Here's how the part is built. I have some questions about the finished solid (model axes, mm). Coordinates: 2 decimals unless noted, no trailing zeros. Loops run counter-clockwise (first coordinate to the right, second up) from the corner with the lowest first, then second, coordinate; pieces in that order, holes last. Notation, with made-up numbers: (53.25, 71) - (79.25, 71) arc R29 ccw to (79.25, 107) - close; hole circle Ø2 at (77, -3). An arc over 180 degrees is marked (long way). Use a Markdown table: item, result.
Autodesk Inventor part; units mm, degrees
ref_plane "YZ Plane" through (0, 0, 0) normal (1, 0, 0) x (0, 1, 0)
ref_plane "XZ Plane" through (0, 0, 0) normal (0, 1, 0) x (-1, 0, 0)
ref_plane "XY Plane" through (0, 0, 0) normal (0, 0, 1) x (1, 0, 0)
sketch "Sketch1" plane through (0, 0, 0) normal (0, 1, 0) x (-1, 0, 0)
  line L0 (25.8082, 8) -> (28.6076, 7.9624) construction
  line L1 (0, 0) -> (0, 92.83)
  line L2 (0, 0) -> (12.1, 0)
  line L3 (26.34, 81.33) -> (8, 81.33)
  line L4 (8, 81.33) -> (8, 32)
  line L5 (8, 32) -> (26.34, 32)
  line L6 (26.34, 32) -> (26.34, 81.33)
  line L7 (0, 92.83) -> (7.42, 92.83)
  line L8 (7.42, 92.83) -> (7.42, 89.33)
  line L9 (7.42, 89.33) -> (26.92, 89.33)
  line L10 (26.92, 89.33) -> (26.92, 92.83)
  line L11 (26.92, 92.83) -> (34.34, 92.83)
  line L12 (34.34, 92.83) -> (34.34, 0)
  line L13 (34.34, 0) -> (12.1, 0)
  line L14 (12.1, 0) -> (12.1, 8)
  line L15 (12.1, 8) -> (34.34, 8)
  spline S0 degree 3 poles (25.8082, 8) (28.6076, 7.9624) (34.5101, 18.742) (34.34, 45.0104) knots 1 1 1 1 1.641396 1.641396 1.641396 1.641396
  line L16 (28.6076, 7.9624) -> (34.5101, 18.742) construction
  line L17 (34.5101, 18.742) -> (34.34, 45.0104) construction
  point P0 (25.8768, 44.3592)
  point P1 (17.17, 89.33)
  point P2 (25.8375, 8)
  point P3 (34.34, 42.8078)
  dimension "d8" = 92.83
  dimension "d9" = 12.1
  dimension "d10" = 7.42
  dimension "d11" = 7.42
  dimension "d12" = 8
  dimension "d13" = 8
  dimension "d14" = 8
  dimension "d15" = 19.5
  dimension "d16" = 3.5
  dimension "d17" = 32
  dimension "d18" = 8
extrude "Extrusion1" add sketch "Sketch1" along normal blind 3 contours L1 L7 L8 L9 L10 L11 L12 S0 L15 L14 L2
properties part number "C-D"
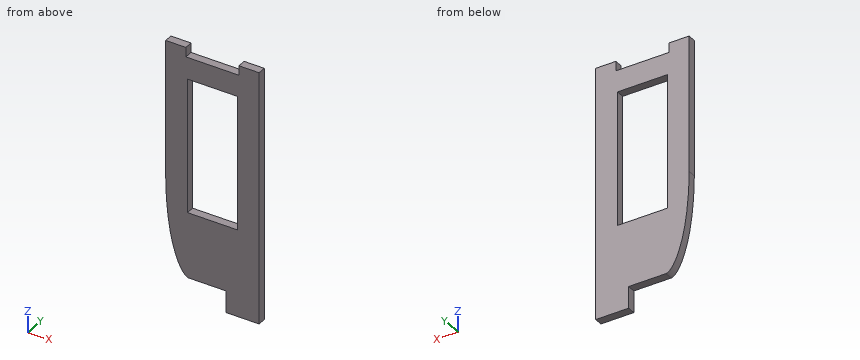
Q1. Please list where these lines run through material, in increasing order: L1, parallel to Z at x = -8.5, y = 0.7; L2, parallel to Z at x = -22.5, y = 1.25; L3, parallel to X at y = 2.5, z = 60. Write a range as from..to.
Check values:
| item | result |
|---|---|
| L1 | 0..32, 81.33..89.33 |
| L2 | 8..32, 81.33..89.33 |
| L3 | -34.34..-26.34, -8..0 |
Q2. I want a section at A-A, the plane x = -16. Write out the boundary of the cut face in (y, z), then the cut area to 3 significant figures.
Check values:
| item | result |
|---|---|
| outline | (0, 8) - (3, 8) - (3, 32) - (0, 32) - close; (0, 81.33) - (3, 81.33) - (3, 89.33) - (0, 89.33) - close |
| area | 96.0 mm^2 |
Q3. Will these pins go through, and if not, where does the flat tip stop? P1, Ø1.5, axis at x = -8.5, z = 56, coming from the -Y side; P2, Ø0.9, axis at x = -12.5, y = 1, coming from the +Z side; P3, Ø0.9, axis at x = -15.5, y = 1.5, coming from the -Z side.
Check values:
| item | result |
|---|---|
| P1 | y = 0 |
| P2 | z = 89.33 |
| P3 | z = 8 |
Q4. I want a section at B-B, the plane z = 59. Write out the boundary of the cut face in (x, y), then the cut area to 3 significant figures.
Check values:
| item | result |
|---|---|
| outline | (-34.34, 0) - (-26.34, 0) - (-26.34, 3) - (-34.34, 3) - close; (-8, 0) - (0, 0) - (0, 3) - (-8, 3) - close |
| area | 48.0 mm^2 |
